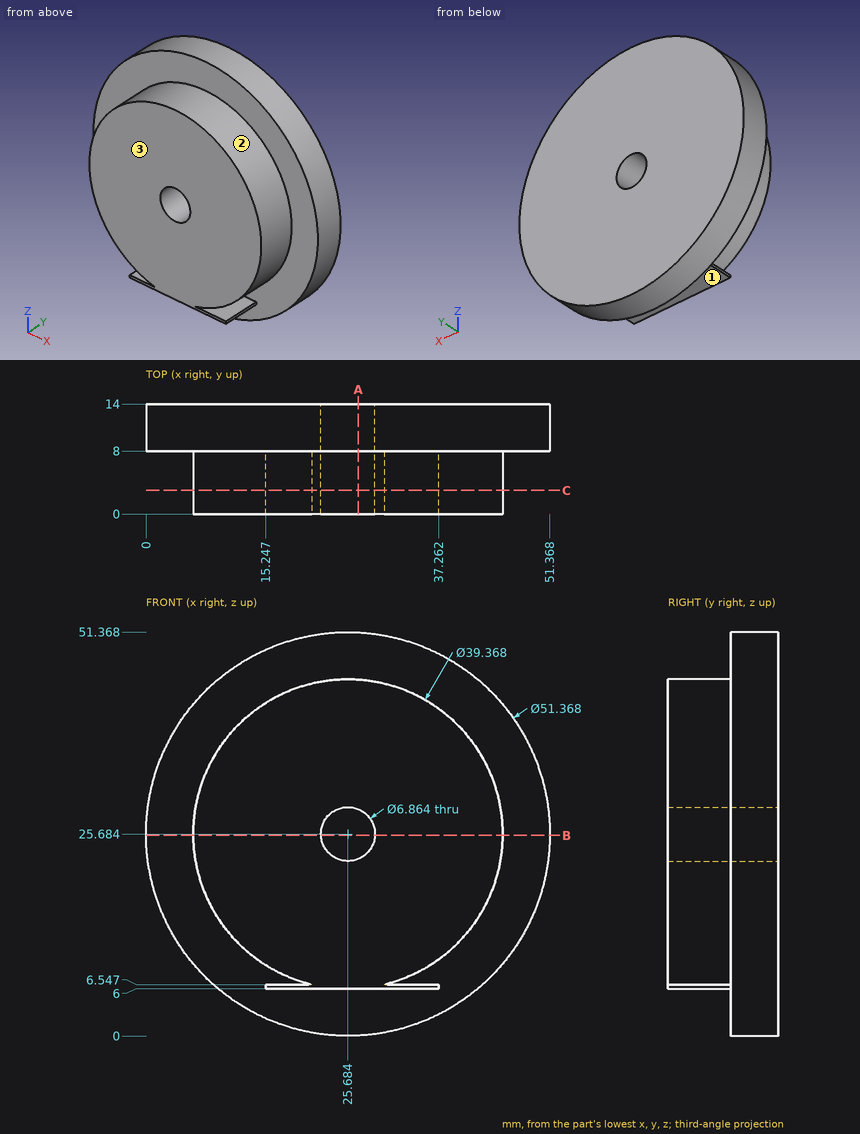
Verification items for this drawing (mm, ordinates from the low corner). Give positions to 0.01 mm unless a question says otherwise; leave off trailing zeros. Write each loop counter-clockwise with the first axis right and the second up, starting at its lowest first coordinate (ties: lowest second). Pieces come first, ordered by that corner, then holes. Notation, with made-up numbers: M -5,25 L 51,25 A24 ccw 51,47 Z; hole C -24,64.5 d3. An arc over 180 degrees is marked long. Use one line per item in the form item = value.
(1) Depth check by flat-ended pin: P1, Ø1.5, axis at x = 16, y = 3, coming from the +Z side (1 decimal); P2, Ø4.5, axis at x = 19, y = 4.5, coming from the +Z side; P3, Ø1.5, axis at y = 10, z = 42, coming from the -X side (1 decimal). Enter the tip coordinate at first touch or a pass-through.
Answer block:
P1 = 43.2
P2 = 44.86
P3 = 5.3
(2) Material ranges on line 1 along Z through (x, y) = (27, 3) (1 decimal); line 2 along Y through (x, z) = (37.5, 8); line 3 along Z through (x, y) = (31, 7.75), recorded low to high.
Answer block:
line_1 = 6 to 22.5, 28.9 to 45.3
line_2 = 8 to 14
line_3 = 6 to 6.55, 6.73 to 44.64
(3) Section check C-C on y = 3. Record the boundary of the cut face in (x, z) (1 decimal), plus the area to 3 significant figures.
Answer block:
outline = M 15.2,6 L 37.3,6 L 37.3,6.5 L 30.3,6.5 A19.7 ccw long 21.1,6.5 L 15.2,6.5 Z; hole C 25.7,25.7 d6.9
area = 1,190 mm2
(4) Section check B-B on z = 25.5. Record the boundary of the cut face in (x, y).
Answer block:
outline = M 0,8 L 6,8 L 6,0 L 22.26,0 L 22.26,14 L 0,14 Z; M 29.11,0 L 45.37,0 L 45.37,8 L 51.37,8 L 51.37,14 L 29.11,14 Z
(5) Draft check along Z on the marked faces 1, 2 and 3. Enter one of: pulls with the +Z half, pulls with the -Z half, needs draft (parallel to the pull), parting line crosses it, or undercut.
Answer block:
face_1 = pulls with the -Z half
face_2 = undercut
face_3 = needs draft
(6) Section check A-A on x = 27. Record the boundary of the cut face in (y, z) (1 decimal), plus the area to 3 significant figures.
Answer block:
outline = M 0,6 L 8,6 L 8,0 L 14,0 L 14,22.5 L 0,22.5 Z; M 0,28.9 L 14,28.9 L 14,51.3 L 8,51.3 L 8,45.3 L 0,45.3 Z
area = 534 mm2
